from build123d import *

# Parameters (mm, degrees)
SKETCH1_W           = 82
SKETCH1_H           = 35
BOSS_EXTRUDE1_DEPTH = 5
SKETCH2_R           = 1.5
CUT_EXTRUDE1_DEPTH  = 4
SKETCH3_R           = 1.5
CUT_EXTRUDE2_DEPTH  = 4
CUT_EXTRUDE3_START  = -4
SKETCH4_R           = 1.5
CUT_EXTRUDE3_DEPTH  = 4


with BuildPart() as part:
    # Sketch1 → Boss-Extrude1 (new body)
    with BuildSketch(Plane(origin=(0, 0, 0), x_dir=(0, 0, -1), z_dir=(1, 0, 0))):
        Rectangle(SKETCH1_W, SKETCH1_H)
    extrude(amount=BOSS_EXTRUDE1_DEPTH)

    # Sketch2 → Cut-Extrude1 (cut)
    with BuildSketch(Plane(origin=(5, 0, 0), x_dir=(0, 0, -1), z_dir=(1, 0, 0))):
        with Locations((-38.5, 9.5)):
            Circle(SKETCH2_R)
        with Locations(Location((-38.5, -9.5, 0), (0, 0, 180))):
            Circle(SKETCH2_R)
        with Locations((38.5, -9.5)):
            Circle(SKETCH2_R)
        with Locations(Location((38.5, 9.5, 0), (0, 0, 180))):
            Circle(SKETCH2_R)
    extrude(amount=-CUT_EXTRUDE1_DEPTH, mode=Mode.SUBTRACT)

    # Sketch3 → Cut-Extrude2 (cut)
    with BuildSketch(Plane.XZ.offset(17.5)):
        with Locations(Location((2.5, 35, 0), (0, 0, 270))):
            Circle(SKETCH3_R)
        with Locations(Location((2.5, -35, 0), (0, 0, 90))):
            Circle(SKETCH3_R)
    extrude(amount=-CUT_EXTRUDE2_DEPTH, mode=Mode.SUBTRACT)

    # Sketch4 → Cut-Extrude3 (cut)
    with BuildSketch(Plane(origin=(0, 17.5, 0), x_dir=(1, 0, 0), z_dir=(0, 1, 0)).offset(CUT_EXTRUDE3_START)):
        with Locations(Location((2.5, -35, 0), (0, 0, 90))):
            Circle(SKETCH4_R)
        with Locations(Location((2.5, 35, 0), (0, 0, 270))):
            Circle(SKETCH4_R)
    extrude(amount=CUT_EXTRUDE3_DEPTH, mode=Mode.SUBTRACT)


solid = part.part
For this review, take the finished solid that the model builds, in its own axes (mm). A direction names the side the tool comes from. Coordinates: 2 decimals unless noted, no trailing zeros. Order: outer loops, then holes, each group sorted by start corner. A loop starts at its lowest first (then second) coordinate and runs counter-clockwise, first axis right, second up. Notation, with made-up numbers: (-19, -33.75) - (35, -33.75) arc R14 cw to (35, -29.75) - close; hole circle Ø10 at (64, 50). An arc over 180 degrees is marked (long way). Use one line per item in the form item = value.
Q1. Consider section C-C (y = -9.5). Give the boundary of the cut face in (x, z), then the cut area to 3 significant figures.
Checked values:
outline = (0, -41) - (5, -41) - (5, -40) - (1, -40) - (1, -37) - (5, -37) - (5, 37) - (1, 37) - (1, 40) - (5, 40) - (5, 41) - (0, 41) - close
area = 386 mm2
Q2. For faces 1 (the flat face through (2, 0, -41)), 2 (the cylindrical face through (3.4, -15.5, -36.2)), 3 (the flat face through (3, 13.5, -35)), 4 (the flat face through (1, -10, 38)), 5 (the flat face through (2, -17.5, 1)), list the 3-axis set-ups (+Z, -Z, +X, -X, +Y, -Y) from which the entire face can be reached by the end or side of a thin tool; tool diameter is ignored.
Checked values:
face_1 = -Z, +X, -X, +Y, -Y
face_2 = -Y
face_3 = +Y
face_4 = +X
face_5 = +Z, -Z, +X, -X, -Y
Q3. For P1, Ø0.9, axis at y = 9.5, z = -38.5, coming from the +X side; P2, Ø2.5, axis at x = 2.5, z = 35, coming from the +Y side; P3, Ø1.5, axis at x = 2, z = -35.5, coming from the -Y side, all flat-tipped, find the tip position at first contact; note any pin that passes through.
Checked values:
P1 = 1
P2 = 13.5
P3 = -13.5
Q4. Draft analysis for pull direction Y (two halves, no side actions). For faces 6 (the flat face through (2, -13.5, -35)), 7 (the cylindrical face through (3.4, 15.5, 36.2)), 8 (the cylindrical face through (3, -10.4, -37.3)), state which applies: +Y half, -Y half, draft (parallel to the pull), parting line (faces both ways), or undercut.
Checked values:
face_6 = -Y half
face_7 = draft
face_8 = undercut
Q5. Consider section B-B (y = 14.5). Give the boundary of the cut face in (x, z), then the cut area to 3 significant figures.
Checked values:
outline = (0, -41) - (5, -41) - (5, 41) - (0, 41) - close; hole circle Ø3 at (2.5, -35); hole circle Ø3 at (2.5, 35)
area = 396 mm2
Q6. Consider section A-A (z = -35). Give the boundary of the cut face in (x, y), then the cut area to 3 significant figures.
Checked values:
outline = (0, -17.5) - (1, -17.5) - (1, -13.5) - (4, -13.5) - (4, -17.5) - (5, -17.5) - (5, 17.5) - (4, 17.5) - (4, 13.5) - (1, 13.5) - (1, 17.5) - (0, 17.5) - close
area = 151 mm2
Q7. For probe 1 along Y at (x, z) = (2, 38.5); probe 2 along X at (y, z) = (-14.5, -35); probe 3 along Z at (x, y) = (3.5, 15.5), list the stretches that pass through material, from the lowest coordinate up. Write a range as from..to.
Checked values:
probe_1 = -17.5..-11, -8..8, 11..17.5
probe_2 = 0..1, 4..5
probe_3 = -41..-36.12, -33.88..33.88, 36.12..41
